from build123d import *

# Parameters (mm, degrees)
F0_W     = 146
F0_H     = 165
F1_DEPTH = 41.7
F2_W     = 148
F2_H     = 42.7
F3_DEPTH = 5
F5_D     = 2.4
F5_DEPTH = 7.8
F5_TIP   = 0.7210327428


with BuildPart() as f1:
    # F0 (on Top) → F1 (new body)
    with BuildSketch(Plane.XY):
        with Locations((73, 82.5)):
            Rectangle(F0_W, F0_H)
    extrude(amount=F1_DEPTH)

    # F2 (on face) → F3 (join)
    with BuildSketch(Plane.XZ):
        with Locations((73, 21.35)):
            Rectangle(F2_W, F2_H)
    extrude(amount=F3_DEPTH)

    # F5
    with Locations(Plane.XY.offset(41.7)):
        with Locations((3.3, 126), (142.7, 126), (142.7, 47), (3.3, 47)):
            Hole(F5_D / 2, depth=F5_DEPTH)
            with Locations((0, 0, -(F5_DEPTH + F5_TIP / 2))):  # 118° drill point
                Cone(0, F5_D / 2, F5_TIP, mode=Mode.SUBTRACT)


solid = f1.part
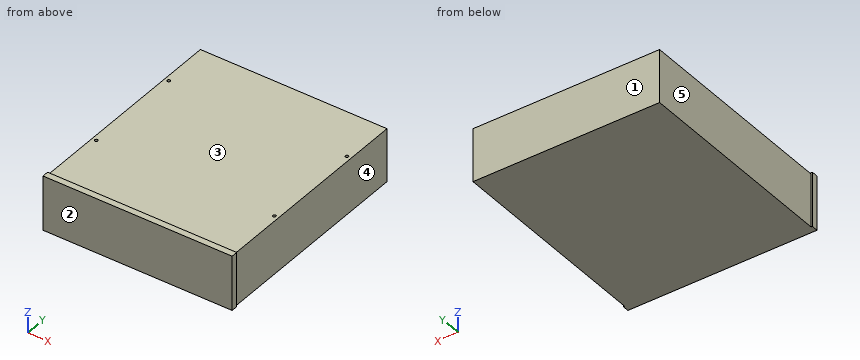
Geometry check sheet. Reference: the model listing, model coordinates, mm. Face numbers are marked on the shaded views. A direction names the side the tool comes from. Give positions to 0.01 mm unless a question says otherwise; leave off trailing zeros. Order: outer loops, then holes, each group sorted by start corner. A loop starts at its lowest first (then second) coordinate and runs counter-clockwise, first axis right, second up. Notation, with made-up numbers: M 30,44 L 54,44 A25 ccw 54,62 Z; hole C 81,13.5 d4. An arc over 180 degrees is marked long. Use a Markdown table: item, result.
Item 1: Section check B-B (y = 37.5). Record the cut outline in (x, z), and give its area (3 significant figures).
Answers follow:
| item | result |
|---|---|
| outline | M 0,0 L 146,0 L 146,41.7 L 0,41.7 Z |
| area | 6,090 mm2 |
Item 2: Section check A-A (x = 125). Record the cut outline in (y, z), and give its area (3 significant figures).
Answers follow:
| item | result |
|---|---|
| outline | M -5,0 L 165,0 L 165,41.7 L 0,41.7 L 0,42.7 L -5,42.7 Z |
| area | 7,090 mm2 |
Item 3: Tool access check on the marked faces 1, 2, 3, 4 and 5. Record the directions out of +Z, -Z, +X, -X, +Y, -Y that give a thin tool (end or side, any length) a straight path to the whole face; none if there is none.
Answers follow:
| item | result |
|---|---|
| face 1 | +Z, -Z, +X, -X, +Y |
| face 2 | +Z, -Z, +X, -X, -Y |
| face 3 | +Z, +X, -X, +Y |
| face 4 | +Z, -Z, +X, +Y |
| face 5 | +Z, -Z, -X, +Y |
Item 4: Depth check by flat-ended pin: P1, Ø1.5, axis at y = 105.5, z = 26.5, coming from the -X side; P2, Ø5, axis at y = 37.5, z = 35, coming from the +X side; P3, Ø4, axis at x = 124, y = 111.5, coming from the +Z side. Enter the tip coordinate at first touch or a pass-through.
Answers follow:
| item | result |
|---|---|
| P1 | stops at x = 0 |
| P2 | stops at x = 146 |
| P3 | stops at z = 41.7 |
Item 5: Material ranges on line 1 along Y through (x, z) = (3, 37); line 2 along X through (y, z) = (126, 38.25); line 3 along Z through (x, y) = (103, 47.5), recorded low to high.
Answers follow:
| item | result |
|---|---|
| line 1 | y = -5 to 45.84, 48.16 to 124.84, 127.16 to 165 |
| line 2 | x = 0 to 2.1, 4.5 to 141.5, 143.9 to 146 |
| line 3 | z = 0 to 41.7 |
